from build123d import *

# Parameters (mm, degrees)
BOSS_EXTRUDE1_DEPTH     = 1.7
CUT_EXTRUDE1_REACH      = 3.7
SKETCH2_R               = 1.1
SKETCH3_R               = 3.43
SKETCH3_R_2             = 2.33
BOSS_EXTRUDE2_DEPTH     = 2.21
SKETCH4_R               = 3.5
SKETCH4_R_2             = 2.95
BOSS_EXTRUDE3_DEPTH     = 0.51
SKETCH5_R               = 2.95
CUT_EXTRUDE2_DEPTH      = 1.1
CUT_EXTRUDE3_REACH      = 4.21
SKETCH6_R               = 0.525
SKETCH7_R               = 18.883041925
SKETCH7_R_2             = 8.25
CUT_EXTRUDE4_DEPTH      = 3.21
CUT_EXTRUDE4_DEPTH_BACK = 3.21


with BuildPart() as part:
    # Sketch1 → Boss-Extrude1 (new body)
    with BuildSketch(Plane.XY):
        with BuildLine():
            Line((5.409077957, 3.736708277), (13.762285951, 2.084772448))
            ThreePointArc((13.762285951, 2.084772448), (15.475148434, 0), (13.762285951, -2.084772448))
            Line((13.762285951, -2.084772448), (5.409077957, -3.736708277))
            ThreePointArc((5.409077957, -3.736708277), (4.318733201, -4.318733201), (3.736708277, -5.409077957))
            Line((3.736708277, -5.409077957), (2.084772448, -13.762285951))
            ThreePointArc((2.084772448, -13.762285951), (0, -15.475148434), (-2.084772448, -13.762285951))
            Line((-2.084772448, -13.762285951), (-3.736708277, -5.409077957))
            ThreePointArc((-3.736708277, -5.409077957), (-4.318733201, -4.318733201), (-5.409077957, -3.736708277))
            Line((-5.409077957, -3.736708277), (-13.762285951, -2.084772448))
            ThreePointArc((-13.762285951, -2.084772448), (-15.475148434, 0), (-13.762285951, 2.084772448))
            Line((-13.762285951, 2.084772448), (-5.409077957, 3.736708277))
            ThreePointArc((-5.409077957, 3.736708277), (-4.318733201, 4.318733201), (-3.736708277, 5.409077957))
            Line((-3.736708277, 5.409077957), (-2.084772448, 13.762285951))
            ThreePointArc((-2.084772448, 13.762285951), (0, 15.475148434), (2.084772448, 13.762285951))
            Line((2.084772448, 13.762285951), (3.736708277, 5.409077957))
            ThreePointArc((3.736708277, 5.409077957), (4.318733201, 4.318733201), (5.409077957, 3.736708277))
        make_face()
    extrude(amount=BOSS_EXTRUDE1_DEPTH)

    # Sketch2 → Cut-Extrude1 (cut, up to next)
    with BuildSketch(Plane.XY.offset(1.7), mode=Mode.PRIVATE) as cut_extrude1_sk1:
        Circle(SKETCH2_R)
    cut_extrude1_tool1 = extrude(cut_extrude1_sk1.sketch, amount=-CUT_EXTRUDE1_REACH, mode=Mode.PRIVATE) & part.part
    add(cut_extrude1_tool1.solids().sort_by_distance((0, 0, 1.7))[0], mode=Mode.SUBTRACT)

    # Sketch3 → Boss-Extrude2 (add)
    with BuildSketch(Plane.XY.offset(1.7)):
        Circle(SKETCH3_R)
        Circle(SKETCH3_R_2, mode=Mode.SUBTRACT)
    extrude(amount=BOSS_EXTRUDE2_DEPTH)

    # Sketch4 → Boss-Extrude3 (add)
    with BuildSketch(Plane(origin=(0, 0, 0), x_dir=(-1, 0, 0), z_dir=(0, 0, -1))):
        Circle(SKETCH4_R)
        Circle(SKETCH4_R_2, mode=Mode.SUBTRACT)
    extrude(amount=BOSS_EXTRUDE3_DEPTH)

    # Sketch5 → Cut-Extrude2 (cut)
    with BuildSketch(Plane(origin=(0, 0, -0.51), x_dir=(-1, 0, 0), z_dir=(0, 0, -1))):
        Circle(SKETCH5_R)
    extrude(amount=-CUT_EXTRUDE2_DEPTH, mode=Mode.SUBTRACT)

    # Sketch6 → Cut-Extrude3 (cut, up to next)
    with BuildSketch(Plane.XY.offset(1.7), mode=Mode.PRIVATE) as cut_extrude3_sk1:
        with Locations((0, 13.35)):
            Circle(SKETCH6_R)
    cut_extrude3_tool1 = extrude(cut_extrude3_sk1.sketch, amount=-CUT_EXTRUDE3_REACH, mode=Mode.PRIVATE) & part.part
    add(cut_extrude3_tool1.solids().sort_by_distance((0, 13.35, 1.7))[0], mode=Mode.SUBTRACT)
    # Sketch6 → Cut-Extrude3 (cut, up to next)
    with BuildSketch(Plane.XY.offset(1.7), mode=Mode.PRIVATE) as cut_extrude3_sk2:
        with Locations((0, 10.6)):
            Circle(SKETCH6_R)
    cut_extrude3_tool2 = extrude(cut_extrude3_sk2.sketch, amount=-CUT_EXTRUDE3_REACH, mode=Mode.PRIVATE) & part.part
    add(cut_extrude3_tool2.solids().sort_by_distance((0, 10.6, 1.7))[0], mode=Mode.SUBTRACT)
    # Sketch6 → Cut-Extrude3 (cut, up to next)
    with BuildSketch(Plane.XY.offset(1.7), mode=Mode.PRIVATE) as cut_extrude3_sk3:
        with Locations((0, 7.85)):
            Circle(SKETCH6_R)
    cut_extrude3_tool3 = extrude(cut_extrude3_sk3.sketch, amount=-CUT_EXTRUDE3_REACH, mode=Mode.PRIVATE) & part.part
    add(cut_extrude3_tool3.solids().sort_by_distance((0, 7.85, 1.7))[0], mode=Mode.SUBTRACT)
    # Sketch6 → Cut-Extrude3 (cut, up to next)
    with BuildSketch(Plane.XY.offset(1.7), mode=Mode.PRIVATE) as cut_extrude3_sk4:
        with Locations((13.35, 0)):
            Circle(SKETCH6_R)
    cut_extrude3_tool4 = extrude(cut_extrude3_sk4.sketch, amount=-CUT_EXTRUDE3_REACH, mode=Mode.PRIVATE) & part.part
    add(cut_extrude3_tool4.solids().sort_by_distance((13.35, 0, 1.7))[0], mode=Mode.SUBTRACT)
    # Sketch6 → Cut-Extrude3 (cut, up to next)
    with BuildSketch(Plane.XY.offset(1.7), mode=Mode.PRIVATE) as cut_extrude3_sk5:
        with Locations((10.6, 0)):
            Circle(SKETCH6_R)
    cut_extrude3_tool5 = extrude(cut_extrude3_sk5.sketch, amount=-CUT_EXTRUDE3_REACH, mode=Mode.PRIVATE) & part.part
    add(cut_extrude3_tool5.solids().sort_by_distance((10.6, 0, 1.7))[0], mode=Mode.SUBTRACT)
    # Sketch6 → Cut-Extrude3 (cut, up to next)
    with BuildSketch(Plane.XY.offset(1.7), mode=Mode.PRIVATE) as cut_extrude3_sk6:
        with Locations((7.85, 0)):
            Circle(SKETCH6_R)
    cut_extrude3_tool6 = extrude(cut_extrude3_sk6.sketch, amount=-CUT_EXTRUDE3_REACH, mode=Mode.PRIVATE) & part.part
    add(cut_extrude3_tool6.solids().sort_by_distance((7.85, 0, 1.7))[0], mode=Mode.SUBTRACT)
    # Sketch6 → Cut-Extrude3 (cut, up to next)
    with BuildSketch(Plane.XY.offset(1.7), mode=Mode.PRIVATE) as cut_extrude3_sk7:
        with Locations((0, -13.35)):
            Circle(SKETCH6_R)
    cut_extrude3_tool7 = extrude(cut_extrude3_sk7.sketch, amount=-CUT_EXTRUDE3_REACH, mode=Mode.PRIVATE) & part.part
    add(cut_extrude3_tool7.solids().sort_by_distance((0, -13.35, 1.7))[0], mode=Mode.SUBTRACT)
    # Sketch6 → Cut-Extrude3 (cut, up to next)
    with BuildSketch(Plane.XY.offset(1.7), mode=Mode.PRIVATE) as cut_extrude3_sk8:
        with Locations((0, -10.6)):
            Circle(SKETCH6_R)
    cut_extrude3_tool8 = extrude(cut_extrude3_sk8.sketch, amount=-CUT_EXTRUDE3_REACH, mode=Mode.PRIVATE) & part.part
    add(cut_extrude3_tool8.solids().sort_by_distance((0, -10.6, 1.7))[0], mode=Mode.SUBTRACT)
    # Sketch6 → Cut-Extrude3 (cut, up to next)
    with BuildSketch(Plane.XY.offset(1.7), mode=Mode.PRIVATE) as cut_extrude3_sk9:
        with Locations((0, -7.85)):
            Circle(SKETCH6_R)
    cut_extrude3_tool9 = extrude(cut_extrude3_sk9.sketch, amount=-CUT_EXTRUDE3_REACH, mode=Mode.PRIVATE) & part.part
    add(cut_extrude3_tool9.solids().sort_by_distance((0, -7.85, 1.7))[0], mode=Mode.SUBTRACT)
    # Sketch6 → Cut-Extrude3 (cut, up to next)
    with BuildSketch(Plane.XY.offset(1.7), mode=Mode.PRIVATE) as cut_extrude3_sk10:
        with Locations((-13.35, 0)):
            Circle(SKETCH6_R)
    cut_extrude3_tool10 = extrude(cut_extrude3_sk10.sketch, amount=-CUT_EXTRUDE3_REACH, mode=Mode.PRIVATE) & part.part
    add(cut_extrude3_tool10.solids().sort_by_distance((-13.35, 0, 1.7))[0], mode=Mode.SUBTRACT)
    # Sketch6 → Cut-Extrude3 (cut, up to next)
    with BuildSketch(Plane.XY.offset(1.7), mode=Mode.PRIVATE) as cut_extrude3_sk11:
        with Locations((-10.6, 0)):
            Circle(SKETCH6_R)
    cut_extrude3_tool11 = extrude(cut_extrude3_sk11.sketch, amount=-CUT_EXTRUDE3_REACH, mode=Mode.PRIVATE) & part.part
    add(cut_extrude3_tool11.solids().sort_by_distance((-10.6, 0, 1.7))[0], mode=Mode.SUBTRACT)
    # Sketch6 → Cut-Extrude3 (cut, up to next)
    with BuildSketch(Plane.XY.offset(1.7), mode=Mode.PRIVATE) as cut_extrude3_sk12:
        with Locations((-7.85, 0)):
            Circle(SKETCH6_R)
    cut_extrude3_tool12 = extrude(cut_extrude3_sk12.sketch, amount=-CUT_EXTRUDE3_REACH, mode=Mode.PRIVATE) & part.part
    add(cut_extrude3_tool12.solids().sort_by_distance((-7.85, 0, 1.7))[0], mode=Mode.SUBTRACT)

    # Sketch7 → Cut-Extrude4 (cut, two sides)
    with BuildSketch(Plane.XY.offset(1.7)) as cut_extrude4_sk:
        Circle(SKETCH7_R)
        Circle(SKETCH7_R_2, mode=Mode.SUBTRACT)
    extrude(amount=CUT_EXTRUDE4_DEPTH, mode=Mode.SUBTRACT)
    extrude(cut_extrude4_sk.sketch, amount=-CUT_EXTRUDE4_DEPTH_BACK, mode=Mode.SUBTRACT)


solid = part.part
Source: CAD feature listing. Evaluate the final solid. Frame: model axes, mm. A direction names the side the tool comes from. Coordinates: 2 decimals unless noted, no trailing zeros. Loops run counter-clockwise (first coordinate to the right, second up) from the corner with the lowest first, then second, coordinate; pieces in that order, holes last. Notation, with made-up numbers: M -10.5,-31.5 L 9.5,-31.5 A21 cw 9.5,4.5 Z; hole C 69.5,77 d4. An arc over 180 degrees is marked long. Answer in a Markdown table with one row per item.
Q1. Section B-B on z = 0.35. Return the cut outline in (x, y) (3 decimals).
Answers below:
| item | result |
|---|---|
| outline | M -8.243,-0.349 A8.25 ccw -7.556,-3.312 L -5.409,-3.737 A2.125 cw -3.737,-5.409 L -3.312,-7.556 A8.25 ccw -0.349,-8.243 A0.525 cw long 0.349,-8.243 A8.25 ccw 3.312,-7.556 L 3.737,-5.409 A2.125 cw 5.409,-3.737 L 7.556,-3.312 A8.25 ccw 8.243,-0.349 A0.525 cw long 8.243,0.349 A8.25 ccw 7.556,3.312 L 5.409,3.737 A2.125 cw 3.737,5.409 L 3.312,7.556 A8.25 ccw 0.349,8.243 A0.525 cw long -0.349,8.243 A8.25 ccw -3.312,7.556 L -3.737,5.409 A2.125 cw -5.409,3.737 L -7.556,3.312 A8.25 ccw -8.243,0.349 A0.525 cw long Z; hole C 0,0 d5.9 |
Q2. Section A-A on y = 0. Return the cut outline in (x, z) (3 decimals).
Answers below:
| item | result |
|---|---|
| outline | M -7.325,0 L -3.5,0 L -3.5,-0.51 L -2.95,-0.51 L -2.95,0.59 L -1.1,0.59 L -1.1,1.7 L -2.33,1.7 L -2.33,3.91 L -3.43,3.91 L -3.43,1.7 L -7.325,1.7 Z; M 1.1,0.59 L 2.95,0.59 L 2.95,-0.51 L 3.5,-0.51 L 3.5,0 L 7.325,0 L 7.325,1.7 L 3.43,1.7 L 3.43,3.91 L 2.33,3.91 L 2.33,1.7 L 1.1,1.7 Z |
Q3. Draft query along X for faces 1 (the flat face through (-6.5, 3.52, 0.84)), 2 (the flat face through (-1, 1, 1.7)), 3 (the cylindrical face through (7.325, 0.018, 0.862)), 4 (the flat face through (-4, 0, 1.7)). Return one class per face: pulls with the +X half, pulls with the -X half, needs draft (parallel to the pull), parting line crosses it, or undercut.
Answers below:
| item | result |
|---|---|
| face 1 | pulls with the -X half |
| face 2 | undercut |
| face 3 | undercut |
| face 4 | needs draft |
Q4. Set-up query: faces 5 (the cylindrical face through (2.947, 0.13, 0.032)), 6 (the cylindrical face through (-1.849, -1.418, 2.79)), 7 (the flat face through (3, -1, -0.51)). Return all of +Z, -Z, +X, -X, +Y, -Y with unobstructed straight access to the full face (end or side cutting, diameter ignored); none if empty.
Answers below:
| item | result |
|---|---|
| face 5 | -Z |
| face 6 | +Z |
| face 7 | -Z, +X, -X, +Y, -Y |
Q5. Ray query, probe 1 along Z at (x, y) = (-4, -3.5); probe 2 along Y at (x, z) = (0, 1.45) (3 decimals); probe 3 along Y at (x, z) = (1, 1.85). Return the intervals inside material, ascending. Write a range as from..to.
Answers below:
| item | result |
|---|---|
| probe 1 | z = 0..1.7 |
| probe 2 | y = -7.325..-1.1, 1.1..7.325 |
| probe 3 | y = -3.28..-2.1, 2.1..3.28 |
Q6. Section D-D on y = 7.85. Return the cut outline in (x, z) (3 decimals), plus the area to 3 significant figures.
Answers below:
| item | result |
|---|---|
| outline | M -2.538,0 L -0.525,0 L -0.525,1.7 L -2.538,1.7 Z; M 0.525,0 L 2.538,0 L 2.538,1.7 L 0.525,1.7 Z |
| area | 6.84 mm^2 |
Q7. First-contact query: pin 1 (6 mm diameter, centred on x = 5.5, y = -3.5, fed in from +Z); pin 2 (2 mm diameter, centred on x = 2, y = -5.5, fed in from -Z); pin 3 (5.5 mm diameter, centred on x = 0, y = 0, fed in from -Z). Flat tips, straight axial feed; report the tip coordinate or a pass-through.
Answers below:
| item | result |
|---|---|
| pin 1 | stops at z = 1.7 |
| pin 2 | stops at z = 0 |
| pin 3 | stops at z = 0.59 |
